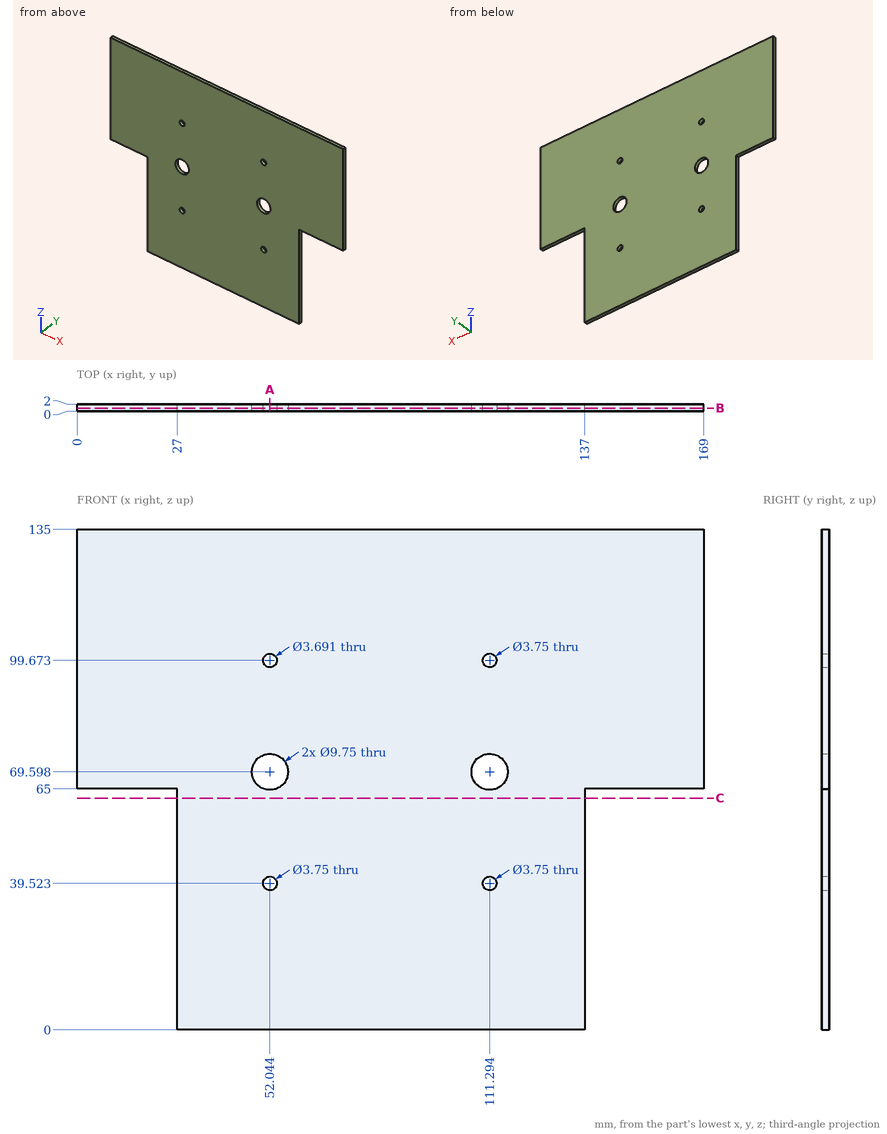
The drawing under review shows one solid part. Ordinate dimensions are in mm from its lowest x, y, z. Give positions to 0.01 mm unless a question says otherwise; leave off trailing zeros. Loops run counter-clockwise (first coordinate to the right, second up) from the corner with the lowest first, then second, coordinate; pieces in that order, holes last. Notation, with made-up numbers: M -23,68.5 L 2,68.5 A19 ccw 2,89.5 Z; hole C -0.5,82.5 d3. An arc over 180 degrees is marked long. Return JSON: item names as keys, results as strings. Group by question number.
Item 1: We need section A-A (x = 52). Give the boundary of the cut face in (y, z).
Item 2: We need section C-C (z = 62.5). Give the boundary of the cut face in (x, y).
Item 3: For probe 1 along X at (y, z) = (1.9, 101) (1 decimal); probe 2 along Z at (x, y) = (51.5, 1.45) (1 decimal); probe 3 along X at (y, z) = (1.6, 59.5), list the stretches that pass through material, from the lowest coordinate up.
Item 4: We need section B-B (y = 0.9). Give the number of separate pieces and of enclosed holes in the cut face, and give its area (3 significant figures).
Item 5: Insertion check: pin 1 Ø1 at (x, y) = (154, 1) entering from -Z; pin 2 Ø0.6 at (y, z) = (1, 20) entering from -X; pin 3 Ø1 at (y, z) = (1.5, 41.5) entering from +X. Each pin has a flat end and moves straight along its axis. Give the tip position at first contact, or say it passes through.
Output:
{
 "1": {"outline": "M 0,0 L 2,0 L 2,37.65 L 0,37.65 Z; M 0,41.4 L 2,41.4 L 2,64.72 L 0,64.72 Z; M 0,74.47 L 2,74.47 L 2,97.83 L 0,97.83 Z; M 0,101.52 L 2,101.52 L 2,135 L 0,135 Z"},
 "2": {"outline": "M 27,0 L 137,0 L 137,2 L 27,2 Z"},
 "3": {"probe 1": "x = 0 to 50.8, 53.3 to 110, 112.6 to 169", "probe 2": "z = 0 to 37.7, 41.3 to 64.8, 74.4 to 97.9, 101.4 to 135", "probe 3": "x = 27 to 137"},
 "4": {"separate pieces": "1", "enclosed holes": "6", "area": "18,800 mm^2"},
 "5": {"pin 1": "stops at z = 65", "pin 2": "stops at x = 27", "pin 3": "stops at x = 137"}
}
